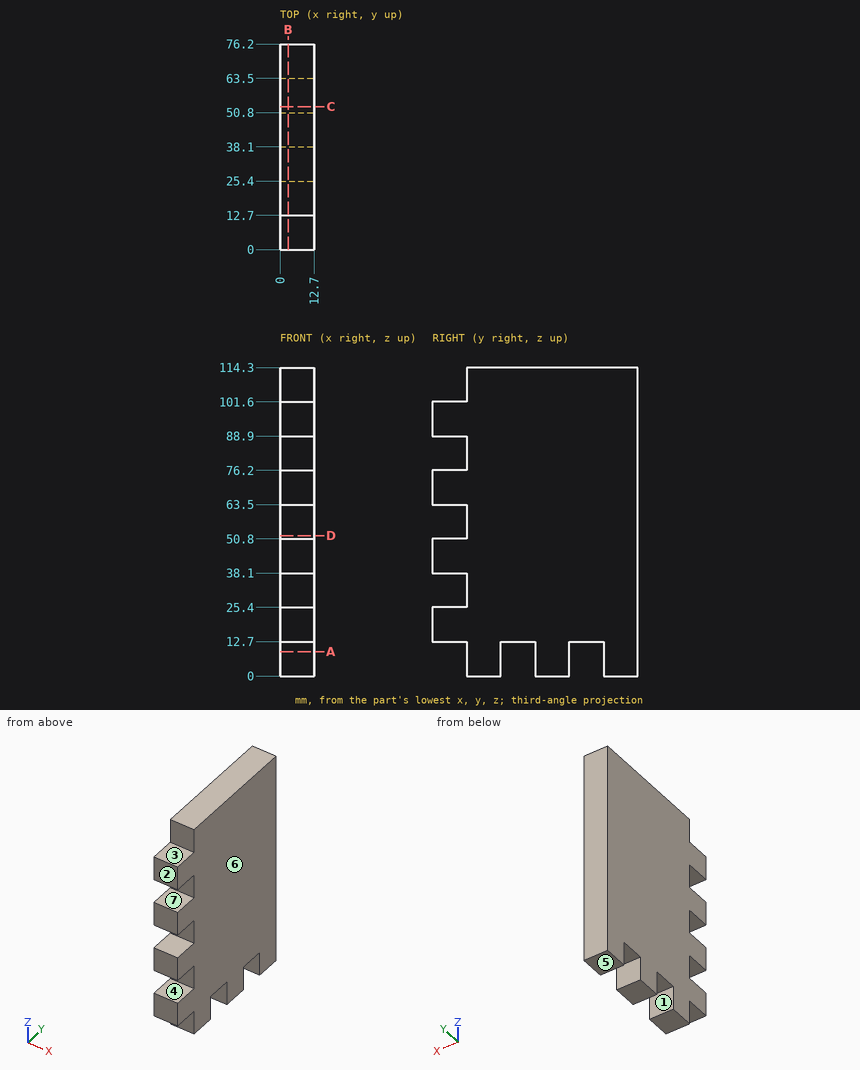
Input: dimensioned drawing with shaded views. Units: mm. Origin: part minimum x, y, z. A direction names the side the tool comes from. Give positions to 0.01 mm unless a question says otherwise; leave off trailing zeros. Write each loop counter-clockwise with the first axis right and the second up, starting at its lowest first coordinate (ties: lowest second). Pieces come first, ordered by that corner, then holes.
1. Section query A-A (z = 9). Return the cut outline in (x, y).
2. Access query for the marked faces 1, 2, 3 and 4. Directions: +Z, -Z, +X, -X, +Y, -Y. A direction counts if a zero-diameter tool reaches every point of the face in a straight line with its end or side. Return the directions, or none.
3. Section query C-C (y = 53). Return the cut outline in (x, z), then the cut area to 3 significant figures.
4. First-contact query: pin 1 (1.5 mm diameter, centred on x = 3.5, z = 57.5, fed in from -Y); pin 2 (4 mm diameter, centred on x = 4.5, y = 3.5, fed in from +Z); pin 3 (6.5 mm diameter, centred on x = 5.5, y = 7.5, fed in from -Z). Flat tips, straight axial feed; report the tip coordinate or a pass-through.
5. Section query D-D (z = 52). Return the cut outline in (x, y), then the cut area to 3 significant figures.
6. Section query B-B (x = 3). Return the cut outline in (y, z), then the cut area to 3 significant figures.
7. Pull-direction query (Z, two-part tool) for the marked faces 5, 6 and 7; classes: +Z half, -Z half, draft (parallel to the pull), parting line (faces both ways), or undercut.
8. Material intervals for line 1 along Y through (x, z) = (1.25, 11); line 2 along Z through (x, y) = (10, 9.5); line 3 along Y through (x, z) = (10.5, 33.5), sorted ascending.
Output values:
1. outline: (0, 12.7) - (12.7, 12.7) - (12.7, 25.4) - (0, 25.4) - close; (0, 38.1) - (12.7, 38.1) - (12.7, 50.8) - (0, 50.8) - close; (0, 63.5) - (12.7, 63.5) - (12.7, 76.2) - (0, 76.2) - close
2. face 1: -Z, +X, -X
2. face 2: +Z, -Z, +X, -X, -Y
2. face 3: +Z, +X, -X, -Y
2. face 4: +X, -X, -Y
3. outline: (0, 12.7) - (12.7, 12.7) - (12.7, 114.3) - (0, 114.3) - close
3. area: 1,290 mm2
4. pin 1: stops at y = 12.7
4. pin 2: stops at z = 101.6
4. pin 3: stops at z = 12.7
5. outline: (0, 12.7) - (12.7, 12.7) - (12.7, 76.2) - (0, 76.2) - close
5. area: 806 mm2
6. outline: (0, 12.7) - (12.7, 12.7) - (12.7, 0) - (25.4, 0) - (25.4, 12.7) - (38.1, 12.7) - (38.1, 0) - (50.8, 0) - (50.8, 12.7) - (63.5, 12.7) - (63.5, 0) - (76.2, 0) - (76.2, 114.3) - (12.7, 114.3) - (12.7, 101.6) - (0, 101.6) - (0, 88.9) - (12.7, 88.9) - (12.7, 76.2) - (0, 76.2) - (0, 63.5) - (12.7, 63.5) - (12.7, 50.8) - (0, 50.8) - (0, 38.1) - (12.7, 38.1) - (12.7, 25.4) - (0, 25.4) - close
6. area: 7,580 mm2
7. face 5: -Z half
7. face 6: draft
7. face 7: undercut
8. line 1: y = 12.7 to 25.4, 38.1 to 50.8, 63.5 to 76.2
8. line 2: z = 12.7 to 25.4, 38.1 to 50.8, 63.5 to 76.2, 88.9 to 101.6
8. line 3: y = 12.7 to 76.2
